The figure shows three views and two pictorial views of one solid part (mm, origin at its lowest corner). Answer the questions. Round coordinates to 2 decimals unless told otherwise and drop trailing zeros. Loops run counter-clockwise (first coordinate to the right, second up) from the corner with the lowest first, then second, coordinate; pieces in that order, holes last. Notation, with made-up numbers: (36, 44.5) -> (90, 44.5) arc R20 ccw to (90, 77.5) -> close; hole circle Ø6 at (7, -8). An arc over 180 degrees is marked (long way). Put each result on its own line as item: value.
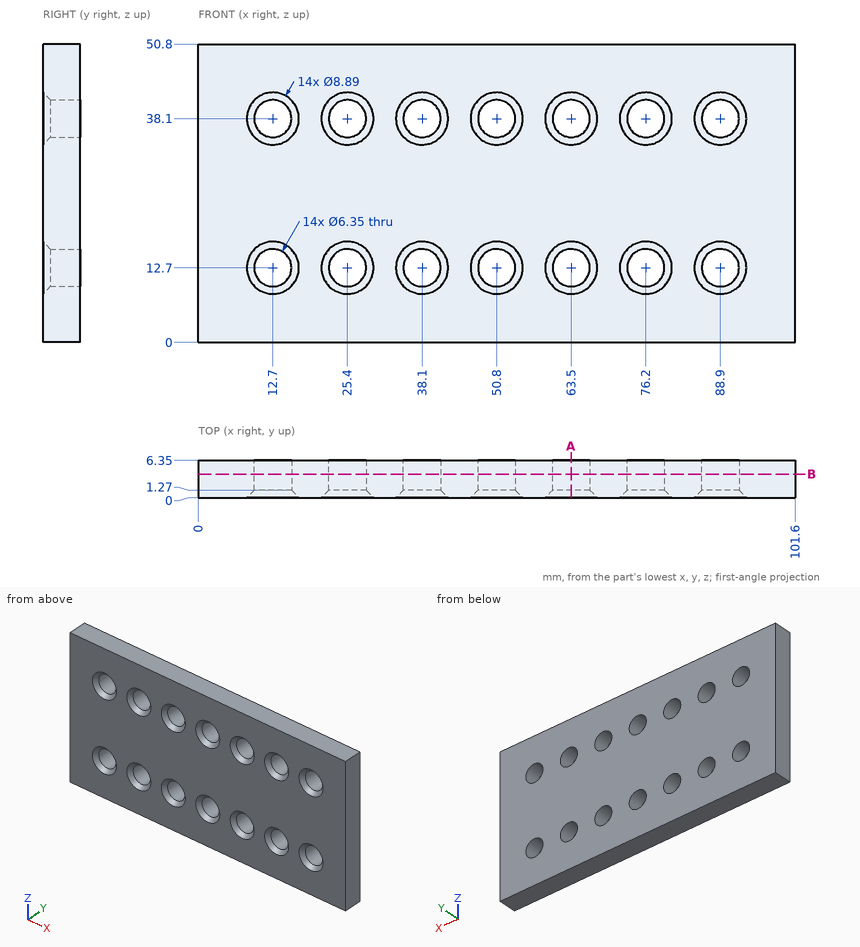
Item 1: Find the intervals of material crossed by line 1 along Z through (x, y) = (38.1, 5.35) (3 decimals); line 2 along Z through (x, y) = (79, 0.5); line 3 along Y through (x, z) = (40, 41), in increasing order.
Derived:
line 1: z = 0 to 9.525, 15.875 to 34.925, 41.275 to 50.8
line 2: z = 0 to 9.92, 15.48 to 35.32, 40.88 to 50.8
line 3: y = 0.98 to 6.35
Item 2: Flat-ended cylindrical pins translate along their axes: pin 1 Ø1 at (x, z) = (78, 9.5) entering from -Y; pin 2 Ø5 at (x, z) = (76.2, 12.7) entering from +Y; pin 3 Ø7.5 at (x, z) = (50.8, 12.7) entering from -Y (3 decimals); pin 4 Ø8.5 at (x, z) = (50.8, 38.1) entering from -Y (3 decimals). Find the tip coordinate at first contact, or state that the pin passes through.
Derived:
pin 1: stops at y = 0.27
pin 2: passes through
pin 3: stops at y = 0.695
pin 4: stops at y = 0.195
Item 3: The part is cut by section A-A (x = 63.5). Determine the outline of the cut face in (y, z) (3 decimals), then the cut area to 3 significant figures.
Derived:
outline: (0, 0) -> (6.35, 0) -> (6.35, 9.525) -> (1.27, 9.525) -> (0, 8.255) -> close; (0, 17.145) -> (1.27, 15.875) -> (6.35, 15.875) -> (6.35, 34.925) -> (1.27, 34.925) -> (0, 33.655) -> close; (0, 42.545) -> (1.27, 41.275) -> (6.35, 41.275) -> (6.35, 50.8) -> (0, 50.8) -> close
area: 239 mm^2
Item 4: The part is cut by section B-B (y = 4). State how many separate pieces and enclosed holes the cut face has, then the cut area to 3 significant figures.
Derived:
separate pieces: 1
enclosed holes: 14
area: 4,720 mm^2
